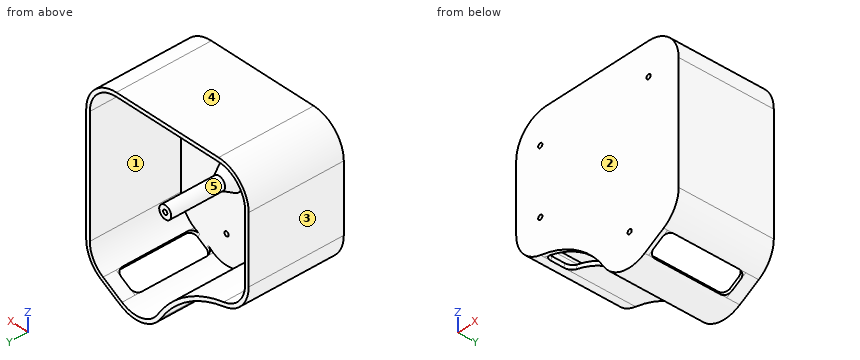
```python
from build123d import *

# Parameters (mm, degrees)
SKETCH1_W           = 260
SKETCH1_H           = 100
BOSS_EXTRUDE1_DEPTH = 3
CUT_EXTRUDE1_DEPTH  = 5
SKETCH5_W           = 260
SKETCH5_H           = 80
BOSS_EXTRUDE4_DEPTH = 3
BOSS_EXTRUDE5_START = 70
BOSS_EXTRUDE5_DEPTH = 70
BOSS_EXTRUDE6_DEPTH = 70
CUT_EXTRUDE3_DEPTH  = 198.810515393
SKETCH10_R          = 5
SKETCH10_R_2        = 1.75
BOSS_EXTRUDE7_DEPTH = 50
CHAMFER1_SIZE       = 5
CHAMFER1_SIZE2      = 8.660254038
FILLET1_R           = 22
FILLET2_R           = 25
CUT_EXTRUDE4_START  = 20
CUT_EXTRUDE4_DEPTH  = 20
SKETCH12_R          = 1.75
CUT_EXTRUDE5_DEPTH  = 20
CUT_EXTRUDE6_DEPTH  = 40
FILLET3_R           = 5


with BuildPart() as part:
    # Sketch1 → Boss-Extrude1 (new body)
    with BuildSketch(Plane(origin=(0, 0, 0), x_dir=(1, 0, 0), z_dir=(0, 1, 0))):
        Rectangle(SKETCH1_W, SKETCH1_H)
    extrude(amount=BOSS_EXTRUDE1_DEPTH)

    # Sketch4 → Cut-Extrude1 (cut)
    with BuildSketch(Plane(origin=(0, 3, 0), x_dir=(1, 0, 0), z_dir=(0, 1, 0))):
        with BuildLine():
            Line((-77.534249575, 30.291115131), (-130, 0))
            Line((-130, 0), (-130, 50))
            Line((-130, 50), (130, 50))
            Line((130, 50), (130, 0))
            Line((130, 0), (77.534249575, 30.291115131))
            ThreePointArc((77.534249575, 30.291115131), (0, -30), (-77.534249575, 30.291115131))
        make_face()
    extrude(amount=-CUT_EXTRUDE1_DEPTH, mode=Mode.SUBTRACT)

    # Sketch5 → Boss-Extrude4 (add)
    with BuildSketch(Plane(origin=(0, 3, 0), x_dir=(1, 0, 0), z_dir=(0, 1, 0))):
        with Locations((0, -90)):
            Rectangle(SKETCH5_W, SKETCH5_H)
    extrude(amount=-BOSS_EXTRUDE4_DEPTH)

    # Sketch6 → Boss-Extrude5 (add)
    with BuildSketch(Plane(origin=(0, 3, 0), x_dir=(1, 0, 0), z_dir=(0, 1, 0)).offset(BOSS_EXTRUDE5_START)):
        with BuildLine():
            Line((-77.534249575, 30.291115131), (-130, 0))
            Line((-130, 0), (-130, -130))
            Line((-130, -130), (130, -130))
            Line((130, -130), (130, 0))
            Line((130, 0), (77.534249575, 30.291115131))
            ThreePointArc((77.534249575, 30.291115131), (0, -30), (-77.534249575, 30.291115131))
        make_face()
        with BuildLine():
            Line((-79.381629809, 25.76042804), (-127, -1.732050808))
            Line((-127, -1.732050808), (-127, -127))
            Line((-127, -127), (127, -127))
            Line((127, -127), (127, -1.732050808))
            Line((127, -1.732050808), (79.381629809, 25.76042804))
            ThreePointArc((79.381629809, 25.76042804), (0, -33), (-79.381629809, 25.76042804))
        make_face(mode=Mode.SUBTRACT)
    extrude(amount=-BOSS_EXTRUDE5_DEPTH)

    # Sketch7 → Boss-Extrude6 (add)
    with BuildSketch(Plane(origin=(0, 73, 0), x_dir=(1, 0, 0), z_dir=(0, 1, 0))):
        with BuildLine():
            Line((-5, -32.849260709), (-5, -130))
            Line((-5, -130), (-2, -130))
            Line((-2, -130), (-2, -32.975900116))
            ThreePointArc((-2, -32.975900116), (-3.500572722, -32.92614781), (-5, -32.849260709))
        make_face()
    extrude(amount=-BOSS_EXTRUDE6_DEPTH)

    # Sketch9 → Cut-Extrude3 (cut, through all)
    with BuildSketch(Plane(origin=(0, 73, 0), x_dir=(1, 0, 0), z_dir=(0, 1, 0))):
        Polygon((-5, -32.849260709), (-5, -144.876678539), (-379.728059333, -144.876678539), (-379.728059333, 52.069032857), (-5, 52.069032857), align=None)
    extrude(amount=-CUT_EXTRUDE3_DEPTH, mode=Mode.SUBTRACT)

    # Sketch10 → Boss-Extrude7 (add)
    # profile 1 of 4: a face of its own
    with BuildSketch(Plane(origin=(0, 3, 0), x_dir=(1, 0, 0), z_dir=(0, 1, 0))):
        with Locations(Location((14, -46.75, 0), (0, 0, 90))):
            Circle(SKETCH10_R)
        with Locations(Location((14, -46.75, 0), (0, 0, 270))):
            Circle(SKETCH10_R_2, mode=Mode.SUBTRACT)
    # profile 2 of 4: a face of its own
    with BuildSketch(Plane(origin=(0, 3, 0), x_dir=(1, 0, 0), z_dir=(0, 1, 0))):
        with Locations(Location((86, -46.75, 0), (0, 0, 90))):
            Circle(SKETCH10_R)
        with Locations(Location((86, -46.75, 0), (0, 0, 270))):
            Circle(SKETCH10_R_2, mode=Mode.SUBTRACT)
    # profile 3 of 4: a face of its own
    with BuildSketch(Plane(origin=(0, 3, 0), x_dir=(1, 0, 0), z_dir=(0, 1, 0))):
        with Locations(Location((86, -113.25, 0), (0, 0, 90))):
            Circle(SKETCH10_R)
        with Locations(Location((86, -113.25, 0), (0, 0, 270))):
            Circle(SKETCH10_R_2, mode=Mode.SUBTRACT)
    # profile 4 of 4: a face of its own
    with BuildSketch(Plane(origin=(0, 3, 0), x_dir=(1, 0, 0), z_dir=(0, 1, 0))):
        with Locations(Location((14, -113.25, 0), (0, 0, 90))):
            Circle(SKETCH10_R)
        with Locations(Location((14, -113.25, 0), (0, 0, 270))):
            Circle(SKETCH10_R_2, mode=Mode.SUBTRACT)
    extrude(amount=BOSS_EXTRUDE7_DEPTH)

    # Chamfer1
    chamfer1_edges = [part.edges().sort_by_distance(p)[0] for p in [
        (86, 3, 51.75),
        (14, 3, 51.75),
        (86, 3, 118.25),
        (14, 3, 118.25),
    ]]
    chamfer1_side = [part.faces().sort_by_distance(p)[0] for p in [
        (68.049806081, 3, 64.998636776),
    ]]
    chamfer(chamfer1_edges, length=CHAMFER1_SIZE, length2=CHAMFER1_SIZE2, reference=chamfer1_side[0])

    # Fillet1
    fillet1_edges = [part.edges().sort_by_distance(p)[0] for p in [
        (-2, 38, 127),
        (-2, 38, 32.975900116),
        (127, 38, 127),
        (127, 38, 1.732050808),
        (79.381629809, 38, -25.76042804),
    ]]
    fillet(fillet1_edges, radius=FILLET1_R)

    # Fillet2
    fillet2_edges = [part.edges().sort_by_distance(p)[0] for p in [
        (-5, 36.5, 29.843597113),
        (-5, 36.5, 130),
        (77.534249575, 36.5, -30.291115131),
        (130, 36.5, 0),
        (130, 36.5, 130),
    ]]
    fillet(fillet2_edges, radius=FILLET2_R)

    # Sketch11 → Cut-Extrude4 (cut)
    with BuildSketch(Plane(origin=(0, 3, 0), x_dir=(1, 0, 0), z_dir=(0, 1, 0)).offset(CUT_EXTRUDE4_START)):
        with BuildLine():
            Line((52.464250206, -10.394556462), (54.431659589, -12.65935233))
            ThreePointArc((54.431659589, -12.65935233), (36.359512028, -24.612236832), (15.80952381, -31.480420697))
            Line((15.80952381, -31.480420697), (15.238095238, -28.53534525))
            ThreePointArc((15.238095238, -28.53534525), (35.045312798, -21.915408995), (52.464250206, -10.394556462))
        make_face()
        Polygon((101.737077009, 16.317606197), (100.237077009, 13.719529986), (116, 4.618802154), (117.5, 7.216878365), align=None)
    extrude(amount=-CUT_EXTRUDE4_DEPTH, mode=Mode.SUBTRACT)

    # Sketch12 → Cut-Extrude5 (cut)
    with BuildSketch(Plane(origin=(0, 3, 0), x_dir=(1, 0, 0), z_dir=(0, 1, 0))):
        with Locations(Location((89.237077009, -5.333028897, 0), (0, 0, 270))):
            Circle(SKETCH12_R)
        with Locations(Location((105, -105, 0), (0, 0, 270))):
            Circle(SKETCH12_R)
        with Locations(Location((15, -105, 0), (0, 0, 66.494954424))):
            Circle(SKETCH12_R)
        with Locations(Location((15, -55, 0), (0, 0, 260.317408662))):
            Circle(SKETCH12_R)
    extrude(amount=-CUT_EXTRUDE5_DEPTH, mode=Mode.SUBTRACT)

    # Sketch14 → Cut-Extrude6 (cut)
    with BuildSketch(Plane.XZ.offset(-23)):
        Polygon((101.737077009, -16.317606197), (117.5, -7.216878365), (116, -4.618802154), (100.237077009, -13.719529986), align=None)
    extrude(amount=-CUT_EXTRUDE6_DEPTH, mode=Mode.SUBTRACT)

    # Fillet3
    # the kernel refuses this fillet: 5 mm, written as the material it adds along each edge
    with BuildSketch(Plane(origin=(101.737077009, 3, -16.317606197), x_dir=(0.8660254037844373, 0, 0.5000000000000024), z_dir=(-0.5000000000000026, 0, 0.8660254037844373))) as fillet3_piece_1_section:
        with BuildLine():
            CenterArc((FILLET3_R, FILLET3_R), FILLET3_R, 180, 90)
            Line((0, FILLET3_R), (0, 0))
            Line((0, 0), (FILLET3_R, 0))
        make_face()
    fillet3_piece_1 = extrude(amount=15.5, mode=Mode.PRIVATE)
    fillet3_piece_1 = fillet3_piece_1 - Plane(origin=(89.237077009, 3.433810283, 5.333028897), x_dir=(-0.8498769238912803, 0, -0.5269812275945843), z_dir=(0, -1, 0)) * Cylinder(22, 52, mode=Mode.PRIVATE)
    add(fillet3_piece_1)
    with BuildSketch(Plane(origin=(109.75, 3, 6.206515394), x_dir=(-0.8660254037844346, 0, -0.500000000000007), z_dir=(0.500000000000007, 0, -0.8660254037844346))) as fillet3_piece_2_section:
        with BuildLine():
            CenterArc((FILLET3_R, FILLET3_R), FILLET3_R, 180, 90)
            Line((0, FILLET3_R), (0, 0))
            Line((0, 0), (FILLET3_R, 0))
        make_face()
    fillet3_piece_2 = extrude(amount=15.5, mode=Mode.PRIVATE)
    fillet3_piece_2 = fillet3_piece_2 - Plane(origin=(105, 4.115508028, 14.43375673), x_dir=(0.5000000000000037, 0, -0.8660254037844366), z_dir=(0, -1, 0)) * Cylinder(22, 51, mode=Mode.PRIVATE)
    add(fillet3_piece_2)
    with BuildSketch(Plane(origin=(44.266711112, 3, 0.957907015), x_dir=(-0.754931955778907, 0, 0.6558031275800951), z_dir=(0.6558031275800951, 0, 0.754931955778907))) as fillet3_piece_3_section:
        with BuildLine():
            CenterArc((FILLET3_R, -FILLET3_R), FILLET3_R, 90, 90)
            Line((0, -FILLET3_R), (0, 0))
            Line((0, 0), (FILLET3_R, 0))
        make_face()
    fillet3_piece_3 = extrude(amount=28, mode=Mode.PRIVATE)
    fillet3_piece_3 = fillet3_piece_3 & Plane(origin=(0, 4.116736713, -50), x_dir=(0.9564051784275456, 0, 0.2920430356590872), z_dir=(0, 1, 0)) * Cylinder(83, 77, mode=Mode.PRIVATE)
    fillet3_piece_3 = fillet3_piece_3 - Plane(origin=(0, 4.116736713, -50), x_dir=(0.9691781196921706, 0, 0.2463610608638238), z_dir=(0, 1, 0)) * Cylinder(80, 77, mode=Mode.PRIVATE)
    add(fillet3_piece_3)
    with BuildSketch(Plane(origin=(18.19047619, 3, 43.751568392), x_dir=(0.9816918156232519, 0, -0.19047619047619338), z_dir=(-0.19047619047619338, 0, -0.981691815623252))) as fillet3_piece_4_section:
        with BuildLine():
            CenterArc((FILLET3_R, -FILLET3_R), FILLET3_R, 90, 90)
            Line((0, -FILLET3_R), (0, 0))
            Line((0, 0), (FILLET3_R, 0))
        make_face()
    fillet3_piece_4 = extrude(amount=28, mode=Mode.PRIVATE)
    fillet3_piece_4 = fillet3_piece_4 - Plane(origin=(20, 4.115502573, 53.07764064), x_dir=(-0.19047619047619013, 0, -0.9816918156232526), z_dir=(0, -1, 0)) * Cylinder(22, 77, mode=Mode.PRIVATE)
    fillet3_piece_4 = fillet3_piece_4 - Plane(origin=(0, 4.115502573, -50), x_dir=(0.9691781196921706, 0, 0.2463610608638238), z_dir=(0, 1, 0)) * Cylinder(80, 77, mode=Mode.PRIVATE)
    add(fillet3_piece_4)
    with BuildSketch(Plane(origin=(44.266711112, 23, 0.957907015), x_dir=(-0.754931955778907, 0, 0.6558031275800951), z_dir=(0.6558031275800951, 0, 0.754931955778907))) as fillet3_piece_5_section:
        with BuildLine():
            CenterArc((FILLET3_R, FILLET3_R), FILLET3_R, 180, 90)
            Line((0, FILLET3_R), (0, 0))
            Line((0, 0), (FILLET3_R, 0))
        make_face()
    fillet3_piece_5 = extrude(amount=28, mode=Mode.PRIVATE)
    fillet3_piece_5 = fillet3_piece_5 & Plane(origin=(0, 21.883263287, -50), x_dir=(0.9564051784275456, 0, 0.2920430356590872), z_dir=(0, 1, 0)) * Cylinder(83, 77, mode=Mode.PRIVATE)
    fillet3_piece_5 = fillet3_piece_5 - Plane(origin=(0, 21.883263287, -50), x_dir=(0.9691781196921706, 0, 0.2463610608638238), z_dir=(0, 1, 0)) * Cylinder(80, 77, mode=Mode.PRIVATE)
    add(fillet3_piece_5)
    with BuildSketch(Plane(origin=(18.19047619, 23, 43.751568392), x_dir=(0, -1, 0), z_dir=(-0.19047619047619338, 0, -0.981691815623252))) as fillet3_piece_6_section:
        with BuildLine():
            CenterArc((FILLET3_R, -FILLET3_R), FILLET3_R, 90, 90)
            Line((0, -FILLET3_R), (0, 0))
            Line((0, 0), (FILLET3_R, 0))
        make_face()
    fillet3_piece_6 = extrude(amount=28, mode=Mode.PRIVATE)
    fillet3_piece_6 = fillet3_piece_6 & Plane(origin=(0, 21.870297326, -50), x_dir=(0.9564051784275456, 0, 0.2920430356590872), z_dir=(0, 1, 0)) * Cylinder(83, 77, mode=Mode.PRIVATE)
    fillet3_piece_6 = fillet3_piece_6 - Plane(origin=(0, 21.870297326, -50), x_dir=(0.9691781196921706, 0, 0.2463610608638238), z_dir=(0, 1, 0)) * Cylinder(80, 77, mode=Mode.PRIVATE)
    add(fillet3_piece_6)
    with BuildSketch(Plane(origin=(100.237077009, 63, -13.719529986), x_dir=(0.866025403784437, 0, 0.5000000000000028), z_dir=(0.5000000000000028, 0, -0.866025403784437))) as fillet3_piece_7:
        with BuildLine():
            CenterArc((FILLET3_R, FILLET3_R), FILLET3_R, 180, 90)
            Line((0, FILLET3_R), (0, 0))
            Line((0, 0), (FILLET3_R, 0))
        make_face()
    extrude(amount=3)
    with BuildSketch(Plane(origin=(117.5, 63, -7.216878365), x_dir=(0, -1, 0), z_dir=(-0.500000000000007, 0, 0.8660254037844346))) as fillet3_piece_8:
        with BuildLine():
            CenterArc((FILLET3_R, -FILLET3_R), FILLET3_R, 90, 90)
            Line((0, -FILLET3_R), (0, 0))
            Line((0, 0), (FILLET3_R, 0))
        make_face()
    extrude(amount=3)


solid = part.part
```
Design review of the part built by this model. Coordinates are the model's own, in mm. Face numbers are marked on the shaded views. A direction names the side the tool comes from. Coordinates: 2 decimals unless noted, no trailing zeros. Order: outer loops, then holes, each group sorted by start corner. A loop starts at its lowest first (then second) coordinate and runs counter-clockwise, first axis right, second up. Notation, with made-up numbers: M -6.5,-1.5 L 26.5,-1.5 A26 ccw 26.5,20.5 Z; hole C 30.25,-35 d3. An arc over 180 degrees is marked long. Answer as a JSON object with one key per item and string values. Group by question number.
1) Add section D-D, the plane x = 29. Write out the cut boundary in (y, z), then the cut area to 3 significant figures.
2) Add section A-A, the plane y = 16. Count the separate pieces of the cut face and the enclosed holes in it, then the cut area to 3 significant figures.
3) For pin 1 (11 mm diameter, centred on x = 84, z = 113.5, fed in from +Y); pin 2 (1 mm diameter, centred on x = 85.5, z = 114, fed in from +Y); pin 3 (3 mm diameter, centred on x = 12, y = 24.5, fed in from +Z), all flat-tipped, find the tip position at first contact; note any pin that passes through.
4) Mouldability with a two-part tool opening along Z and no side actions: class the marked faces 3, 4 and 5 as pulls with the +Z half, pulls with the -Z half, needs draft (parallel to the pull), parting line crosses it, or undercut.
5) Tool access review of the marked faces 1 and 2: name each direction out of +Z, -Z, +X, -X, +Y, -Y from which nothing blocks a thin tool from reaching the whole face with its end or side.
6) Wall thickness on L1, parallel to X at y = 0.8, z = 105; L2, parallel to X at y = 16, z = 95.5; L3, parallel to Z at x = 81.5, y = 21: over which ranges is each line inside the solid? List them lowest first.
7) Add section C-C, the plane z = 25.5. Write out the cut boundary in (x, y), then the cut area to 3 significant figures.
Computed values:
{
 "1": {"outline": "M 0,24.56 L 3,24.56 L 3,127 L 73,127 L 73,130 L 0,130 Z; M 23,24.56 L 73,24.56 L 73,27.77 L 23,27.77 Z", "area": "687 mm^2"},
 "2": {"separate pieces": "6", "enclosed holes": "4", "area": "1,530 mm^2"},
 "3": {"pin 1": "stops at y = 53", "pin 2": "stops at y = 3", "pin 3": "stops at z = 129.14"},
 "4": {"face 3": "needs draft", "face 4": "pulls with the +Z half", "face 5": "undercut"},
 "5": {"face 1": "+Y", "face 2": "+Z, -Z, +X, -X, -Y"},
 "6": {"L1": "x = -5 to 13.25, 16.75 to 103.25, 106.75 to 130", "L2": "x = -5 to -2, 127 to 130", "L3": "z = -18.44 to -15.26, 44.57 to 48.93, 111.07 to 115.43, 127 to 130"},
 "7": {"outline": "M 26.45,0 L 130,0 L 130,73 L 127,73 L 127,3 L 26.45,3 Z; M 26.45,23 L 34.48,23 L 34.48,73 L 26.45,73 Z", "area": "922 mm^2"}
}
